Autodesk Inventor part; units mm, degrees
ref_plane "YZ Plane" through (0, 0, 0) normal (1, 0, 0) x (0, 1, 0)
ref_plane "XZ Plane" through (0, 0, 0) normal (0, 1, 0) x (-1, 0, 0)
ref_plane "XY Plane" through (0, 0, 0) normal (0, 0, 1) x (1, 0, 0)
sketch "Sketch1" plane through (0, 0, 0) normal (0, 1, 0) x (-1, 0, 0)
  line L0 (-50, 4) -> (50, 4)
  line L1 (50, 4) -> (50, -4)
  line L2 (50, -4) -> (-50, -4)
  line L3 (-50, -4) -> (-50, 4)
  line L4 (-50, 4) -> (50, -4) construction
  line L5 (50, 4) -> (-50, -4) construction
  point P0 (0, 0)
  dimension "d0" = 100
  dimension "d1" = 8
extrude "Plate1" add sketch "Sketch1" along normal blind 1.5
sketch "Sketch2" plane through (50, 363.5, 366) normal (0, 0, 1) x (1, 0, 0)
  line L0 (-100, 0) -> (0, 0)
  line L1 (0, 0) -> (0, 8)
  line L2 (0, 8) -> (-100, 8)
  line L3 (-100, 8) -> (-100, 0)
edge flange "Flange1" height 370 angle 90 thickness 1.5 bend radius 362 thickness toward (0, 0, 1) relief tear relief width 1.5 relief depth 0.75 edges at (0, 1.5, 4) wall of the first edge with corners at (-50, 363.5, 366) (50, 363.5, 366) (50, 371.5, 366) (-50, 371.5, 366)
bend "Bend1"
corner "Corner1"
equation "\"d2\" = Thickness"
equation "\"d3\" = BendReliefWidth"
equation "\"d4\" = BendReliefDepth"
equation "\"d5\" = MinimumRemnant"
equation "\"d6\" = TransitionRadius"
equation "\"d10\" = CornerReliefSize"
equation "\"d11\" = GapSize"
equation "\"d12\" = JacobiRadiusSize"
equation "\"BendRadius\" = Thickness"
equation "\"BendReliefWidth\" = Thickness"
equation "\"BendReliefDepth\" = 0.5 * Thickness"
equation "\"CornerReliefSize\" = 4 * Thickness"
equation "\"MinimumRemnant\" = 2 * Thickness"
equation "\"TransitionRadius\" = BendRadius"
equation "\"JacobiRadiusSize\" = BendRadius"
equation "\"GapSize\" = Thickness"
properties part number "CHAPA_8" material "Steel, Mild, Welded"
The model under review builds one solid part; all positions refer to its coordinate system, in mm. Round coordinates to 2 decimals unless told otherwise and drop trailing zeros. Loops run counter-clockwise (first coordinate to the right, second up) from the corner with the lowest first, then second, coordinate; pieces in that order, holes last. Notation, with made-up numbers: (88.5, 67.25) - (111.5, 67.25) arc R10 cw to (111.5, 84.25) - close; hole circle Ø9 at (56, -34). An arc over 180 degrees is marked (long way). Write each question's results on one line, items separated by ' | '. Start each with the question number.
Q1. Take a section at B-B on z = 220.5. Give the boundary of the cut face in (x, y).
Q2. Insertion check: P1, Ø4, axis at x = -13.5, z = -0.5, coming from the +Y side; P2, Ø2, axis at x = -22.5, z = 171, coming from the +Y side; P3, Ø8, axis at x = -1, z = 175.5, coming from the -Y side. Each pin has a flat end and moves straight along its axis. Give the tip position at first contact, or say it passes through.
Q3. Wall thickness on line 1 along Y through (x, z) = (41, 185.5); line 2 along Z through (x, y) = (-29.5, 64.5); line 3 along Z through (x, y) = (-24, 348.5): over which ranges is each line inside the solid? List them lowest first. Write a range as [from, to].
Q4. Take a section at C-C on y = 139. Give the boundary of the cut face in (x, z), plus the area to 3 significant figures.
Q5. Take a section at A-A on x = -1. Give the boundary of the cut face in (y, z).
Data:
1) outline: (-50, 71.51) - (50, 71.51) - (50, 73.38) - (-50, 73.38) - close
2) P1: stops at y = 1.5 | P2: stops at y = 42.84 | P3: stops at y = 40.89
3) line 1: y = [48.56, 50.29] | line 2: z = [208.07, 210.72] | line 3: z = [365.69, 367.19]
4) outline: (-50, 287.98) - (50, 287.98) - (50, 289.89) - (-50, 289.89) - close | area: 191 mm²
5) outline: (0, -4) - (1.5, -4) - (1.5, 4) arc R362 cw to (363.5, 366) - (371.5, 366) - (371.5, 367.5) - (363.5, 367.5) arc R363.5 ccw to (0, 4) - close
